Autodesk Inventor part; units mm, degrees
ref_plane "YZ Plane" through (0, 0, 0) normal (1, 0, 0) x (0, 1, 0)
ref_plane "XZ Plane" through (0, 0, 0) normal (0, 1, 0) x (-1, 0, 0)
ref_plane "XY Plane" through (0, 0, 0) normal (0, 0, 1) x (1, 0, 0)
sketch "Sketch1" plane through (0, 0, 0) normal (0, 0, 1) x (1, 0, 0)
  line L0 (-31.75, 31.75) -> (31.75, 31.75)
  line L1 (31.75, 31.75) -> (31.75, -31.75)
  line L2 (31.75, -31.75) -> (-31.75, -31.75)
  line L3 (-31.75, -31.75) -> (-31.75, 31.75)
  line L4 (0, 0) -> (0, 31.75) construction
  line L5 (0, 0) -> (0, -31.75) construction
  line L6 (0, 0) -> (31.75, 0) construction
  line L7 (0, 0) -> (-31.75, 0) construction
  dimension "d0" = 63.5
  dimension "d1" = 63.5
extrude "Extrusion1" add sketch "Sketch1" along normal mid plane 12.7
sketch "Sketch9" plane through (-31.75, -31.75, 6.35) normal (0, -1, 0) x (1, 0, 0)
  line L0 (63.5, 0) -> (0, 0)
  line L1 (0, 0) -> (0, -12.7)
  line L2 (0, -12.7) -> (63.5, -12.7)
  line L3 (63.5, 0) -> (63.5, -12.7)
  line L4 (0, -6.35) -> (63.5, -6.35) construction
  line L5 (31.75, 0) -> (31.75, -12.7) construction
  point P0 (13.75, -6.35)
  dimension "d37" = 18
hole "Hole3" at (-18, -31.75, 0) direction (0, 1, 0) diameter 4.978 depth 13.7 tip angle 118
sketch "Sketch12" plane through (0, 0, 6.35) normal (0, 0, 1) x (1, 0, 0)
  point P0 (0, 0)
  point P1 (0, 0)
hole "Hole6" at (0, 0, 6.35) direction (0, 0, -1) diameter 13.7 end through all counterbore diameter 21.9964 counterbore depth 10
mirror "Mirror1" about plane through (0, 0, 0) normal (1, 0, 0) of "Hole3"
mirror "Mirror2" about plane through (0, 0, 0) normal (0, 1, 0) of "Hole3", "Mirror1"
chamfer "Chamfer2" distance 1 angle 45 4 edges at (-18, -31.75, 2.489) (18, -31.75, 2.489) (-18, 31.75, 2.489) (18, 31.75, 2.489)
sketch "Sketch11" plane through (0, 0, 6.35) normal (0, 0, 1) x (1, 0, 0)
  circle A0 centre (0, 0) radius 10.9982
  line L0 (31.75, 31.75) -> (31.75, -31.75)
  line L1 (0, 0) -> (31.75, 0) construction
  point P0 (26.9875, 0)
  dimension "d82" = 26.9875
hole "Hole5" at (26.9875, 0, 6.35) direction (0, 0, -1) diameter 4.134 end through all
pattern_circular "Circular Pattern4" count 4 over 360 about axis through (0, 0, -84.3461) along (0, 0, 1) of "Hole5"
chamfer "Chamfer3" distance 0.25 angle 45 8 edges at (26.9875, 2.067, 6.35) (-2.067, 26.9875, 6.35) (-26.9875, -2.067, 6.35) (2.067, -26.9875, 6.35) (-2.067, 26.9875, -6.35) (2.067, -26.9875, -6.35) (-26.9875, -2.067, -6.35) (26.9875, 2.067, -6.35)
properties part number "BB2-FrontPlate" material "Aluminum-6061-AHC"
Verification items for the finished model (mm, model axes). A direction names the side the tool comes from. Give positions to 0.01 mm unless a question says otherwise; leave off trailing zeros. Loops run counter-clockwise (first coordinate to the right, second up) from the corner with the lowest first, then second, coordinate; pieces in that order, holes last.
1. Section check C-C, the plane z = 4.25. Enter the section's corners in (x, y).
2. Mould release check, pull along Y, two halves, no side actions. Record for faces 4 (the flat face through (-31.75, 0, 0)), 5 (the conical face through (18.4, -16.8, 0.1)), 6 (the cylindrical face through (1.111, 25.245, -0.085)), 7 (the conical face through (17.6, 16.8, 0.1)): released by +Y, released by -Y, zero draft, split by the parting line, or undercut.
3. Go/stop test with flat-tipped pins: pin 1 Ø3 at (x, z) = (18, 0) entering from +Y; pin 2 Ø6.5 at (x, z) = (18, 0) entering from +Y; pin 3 Ø8 at (x, y) = (0, 0) entering from +Z; pin 4 Ø11 at (x, y) = (1, 3) entering from +Z. Record where each tip stops, or that it passes through.
4. Set-up check for faces 1 (the cylindrical face through (15.53, -24.31, 0.32)), 2 (the cylindrical face through (20.099, 24.311, -1.338)), 3 (the flat face through (31.75, 0, 0)): record each of +Z, -Z, +X, -X, +Y, -Y from which the full face is reachable in a straight line by a thin tool's end or side.
5. Section check A-A, the plane x = 0. Enter the section's corners in (y, z).
6. Thickness scan on line 1 (Y direction, x = 0, z = 1.5); line 2 (X direction, y = -22.5, z = 0); line 3 (Y direction, x = 0, z = -5.35). Record the ranges inside material, lowest first.
Geometry says:
1. outline: (-31.75, -31.75) - (31.75, -31.75) - (31.75, 31.75) - (-31.75, 31.75) - close; hole circle Ø4.13 at (-26.99, 0); hole circle Ø22 at (0, 0); hole circle Ø4.13 at (0, -26.99); hole circle Ø4.13 at (0, 26.99); hole circle Ø4.13 at (26.99, 0)
2. face 4: zero draft
2. face 5: released by -Y
2. face 6: undercut
2. face 7: released by +Y
3. pin 1: stops at y = 17.46
3. pin 2: stops at y = 31.51
3. pin 3: passes through
3. pin 4: stops at z = -3.65
4. face 1: -Y
4. face 2: +Y
4. face 3: +Z, -Z, +X, +Y, -Y
5. outline: (-31.75, -6.35) - (-29.3, -6.35) - (-29.05, -6.1) - (-29.05, 6.1) - (-29.3, 6.35) - (-31.75, 6.35) - close; (-24.92, -6.1) - (-24.67, -6.35) - (-6.85, -6.35) - (-6.85, -3.65) - (-11, -3.65) - (-11, 6.35) - (-24.67, 6.35) - (-24.92, 6.1) - close; (6.85, -6.35) - (24.67, -6.35) - (24.92, -6.1) - (24.92, 6.1) - (24.67, 6.35) - (11, 6.35) - (11, -3.65) - (6.85, -3.65) - close; (29.05, -6.1) - (29.3, -6.35) - (31.75, -6.35) - (31.75, 6.35) - (29.3, 6.35) - (29.05, 6.1) - close
6. line 1: y = -31.75 to -29.05, -24.92 to -11, 11 to 24.92, 29.05 to 31.75
6. line 2: x = -31.75 to -20.49, -15.51 to 15.51, 20.49 to 31.75
6. line 3: y = -31.75 to -29.05, -24.92 to -6.85, 6.85 to 24.92, 29.05 to 31.75
